Geometry: see drawing. Coordinates: mm, zero at the bounding-box minimum. A direction names the side the tool comes from. Give positions to 0.01 mm unless a question says otherwise; leave off trailing zeros. Write each loop counter-clockwise with the first axis right and the second up, starting at its lowest first coordinate (ties: lowest second). Pieces come first, ordered by that corner, then holes. Notation, with made-up numbers: M -39.5,5.25 L -29.5,5.25 A19 ccw -29.5,23.25 Z; hole C 25,-6.75 d1. An arc over 180 degrees is marked long. Use a Markdown table: item, result. Add a question column.
(1) Draft query along X for the marked faces 1, 2, 3 and 4. Return one class per face: released by +X, released by -X, zero draft, split by the parting line, or undercut.
(2) Reachability of the marked faces 5 and 6 from +Z, -Z, +X, -X, +Y, -Y: full face, straight path, thin tool, end or side. Return the list, or none.
(3) Pin query (flat end, axial travel): pin 1 Ø3 at (y, z) = (1, 7) entering from +X; pin 2 Ø3 at (x, z) = (5, 3) entering from -Y; pin 3 Ø4 at (y, z) = (1, 6) entering from +X. Return the tip coordinate at first contact, or that it passes through.
(4) Material intervals for L1, parallel to Z at x = 3.5, y = 3.75; L2, parallel to X at y = 4.5, z = 4.5 (1 decimal); L3, parallel to Y at x = 3.75, z = 9.5 (1 decimal), sorted ascending.
(5) Cut plane A-A (z = 9). Output: boundary loops of the cut face in (x, y) (1 decimal), plus the area to 3 significant figures.
(6) Cut plane D-D (z = 3.75). Output: boundary loops of the cut face in (x, y) (1 decimal), plus the area to 3 significant figures.
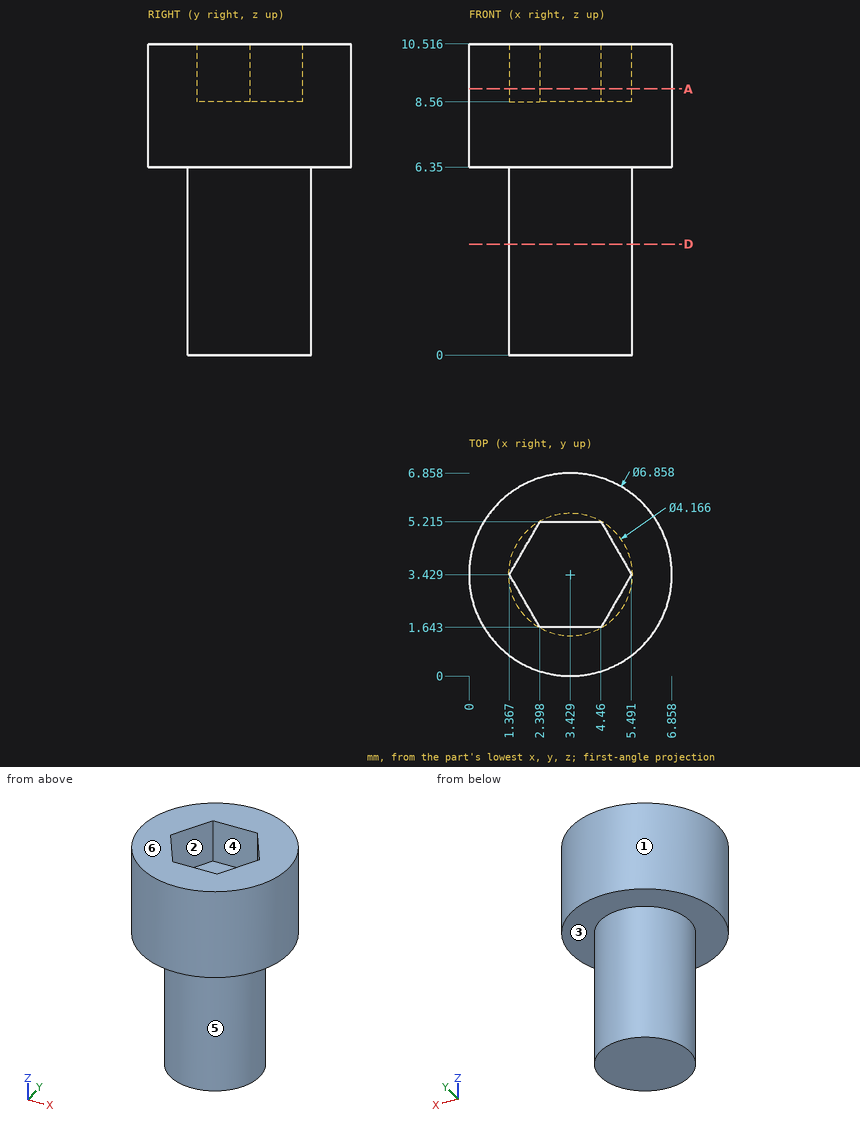
Answer list:
| question | item | result |
|---|---|---|
| 1 | face 1 | split by the parting line |
| 1 | face 2 | undercut |
| 1 | face 3 | zero draft |
| 1 | face 4 | undercut |
| 2 | face 5 | -Z |
| 2 | face 6 | +Z, +X, -X, +Y, -Y |
| 3 | pin 1 | x = 6.73 |
| 3 | pin 2 | y = 1.35 |
| 3 | pin 3 | x = 6.83 |
| 4 | L1 | 0 to 8.56 |
| 4 | L2 | 1.6 to 5.2 |
| 4 | L3 | 0 to 1.6, 5.2 to 6.8 |
| 5 | outline | C 3.4,3.4 d6.9; hole M 1.4,3.4 L 2.4,1.6 L 4.5,1.6 L 5.5,3.4 L 4.5,5.2 L 2.4,5.2 Z |
| 5 | area | 25.9 mm² |
| 6 | outline | C 3.4,3.4 d4.2 |
| 6 | area | 13.6 mm² |
